Geometry: final body of the model. Coordinates: model frame, mm. Face numbers are marked on the shaded views. A direction names the side the tool comes from. Give positions to 0.01 mm unless a question says otherwise; leave off trailing zeros. Loops run counter-clockwise (first coordinate to the right, second up) from the corner with the lowest first, then second, coordinate; pieces in that order, holes last.
1. Section C-C, the plane x = -1.5. Output: boundary loops of the cut face in (y, z) (3 decimals), then the cut area to 3 significant figures.
2. Draft query along X for the marked faces 1, 2, 3 and 4. Return one class per face: +X half, -X half, draft (parallel to the pull), parting line (faces both ways), or undercut.
3. Access query for the marked faces 5, 6 and 7. Directions: +Z, -Z, +X, -X, +Y, -Y. A direction counts if a zero-diameter tool reaches every point of the face in a straight line with its end or side. Return the directions, or none.
4. Section D-D, the plane z = -3.25. Output: boundary loops of the cut face in (x, y) (3 decimals).
5. First-contact query: P1, Ø1, axis at x = -6, y = 3.5, coming from the -Z side; P2, Ø1, axis at y = 3.5, z = -7.5, coming from the -X side; P3, Ø2, axis at x = -1, z = -7, coming from the +Y side; P4, Ø0.5, axis at x = -5, z = -0.5, coming from the +Y side. Flat tips, straight axial feed; report the tip coordinate or a pass-through.
6. Section B-B, the plane z = -7.75. Output: boundary loops of the cut face in (x, y).
7. Material intervals for line 1 along Z through (x, y) = (-5.25, 4.5); line 2 along X through (y, z) = (1.85, -9.25); line 3 along X through (y, z) = (0.3, -9), sorted ascending.
8. Section A-A, the plane y = 4.5. Output: boundary loops of the cut face in (x, z).
Autodesk Inventor part; units mm, degrees
ref_plane "YZ Plane" through (0, 0, 0) normal (1, 0, 0) x (0, 1, 0)
ref_plane "XZ Plane" through (0, 0, 0) normal (0, 1, 0) x (-1, 0, 0)
ref_plane "XY Plane" through (0, 0, 0) normal (0, 0, 1) x (1, 0, 0)
sketch "Sketch1" plane through (0, 0, 0) normal (0, 1, 0) x (-1, 0, 0)
  line L0 (0, 0) -> (8.89, 0)
  line L1 (8.89, 0) -> (8.89, -10.16)
  line L2 (8.89, -10.16) -> (0, -10.16)
  line L3 (0, -10.16) -> (0, 0)
  dimension "d0" = 8.89
  dimension "d1" = 10.16
extrude "Extrusion1" add sketch "Sketch1" along normal blind 2.54
sketch "Sketch5" plane through (0, 2.54, 0) normal (0, 1, 0) x (1, 0, 0)
  line L0 (-8.89, 0) -> (0, 0)
  line L1 (0, 0) -> (0, 10.16)
  line L2 (0, 10.16) -> (-8.89, 10.16)
  line L3 (-8.89, 10.16) -> (-8.89, 0)
  line L4 (0, 0) -> (-8.89, 0)
  line L5 (-5.7785, 0) -> (-6.6294, 0.9271)
  line L6 (-6.6294, 0.9271) -> (-6.6294, 1.6764)
  line L7 (-6.6294, 1.6764) -> (-2.2606, 1.6764)
  line L8 (-2.2606, 1.6764) -> (-2.2606, 0.9271)
  line L9 (-2.2606, 0.9271) -> (-3.1115, 0)
  line L10 (-8.89, 0) -> (-8.89, 10.16)
  line L11 (-8.89, 3.81) -> (0, 3.81)
  point P0 (-4.445, 1.6764)
  point P1 (-4.445, 3.81)
  dimension "d19" = 2.667
  dimension "d20" = 4.3688
  dimension "d21" = 0.9271
  dimension "d23" = 1.6764
  dimension "d24" = 3.81
extrude "Extrusion4" add sketch "Sketch5" along normal blind 3.175 contours L3 L11 L1 L0 L9 L8 L7 L6 L5
sketch "Sketch6" plane through (0, 2.54, 0) normal (0, 1, 0) x (1, 0, 0)
  line L0 (-3.1115, 0) -> (-2.2606, 0.9271)
  line L1 (-2.2606, 0.9271) -> (-2.2606, 1.6764)
  line L2 (-2.2606, 1.6764) -> (-6.6294, 1.6764)
  line L3 (-6.6294, 1.6764) -> (-6.6294, 0.9271)
  line L4 (-6.6294, 0.9271) -> (-5.7785, 0)
  line L5 (-5.7785, 0) -> (-3.1115, 0)
  point P0 (0, 0)
extrude "Extrusion5" cut sketch "Sketch6" against normal blind 1.016
fillet "Fillet3" radius 1.27 6 edges at (-8.89, 1.27, -10.16) (0, 1.27, -10.16) (-8.89, 2.8575, 0) (-8.89, 4.1275, -3.81) (0, 4.1275, -3.81) (0, 2.8575, 0)
sketch "Sketch8" plane through (0, 2.54, 0) normal (0, 1, 0) x (1, 0, 0)
  line L0 (-7.62, 10.16) -> (-1.27, 10.16)
  line L1 (-6.1595, 10.16) -> (-6.1595, 7.874)
  line L2 (-2.7305, 10.16) -> (-2.7305, 7.874)
  arc A0 (-6.1595, 7.874) -> (-2.7305, 7.874) centre (-4.445, 7.874) ccw
  point P0 (0, 0)
  point P1 (-4.445, 10.16)
  dimension "d37" = 3.429
  dimension "d38" = 2.286
extrude "Extrusion7" cut sketch "Sketch8" against normal blind 25.4
fillet "Fillet4" radius 1.016 2 edges at (-2.7305, 1.27, -10.16) (-6.1595, 1.27, -10.16)
properties part number "HallEffectSpoolSensorMount3" material "ABS Plastic"
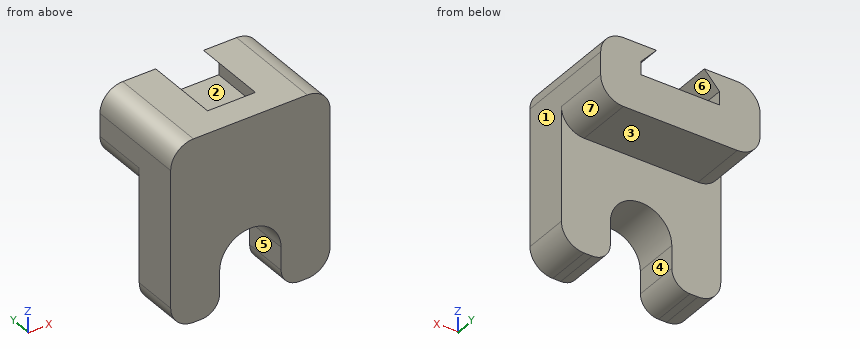
Answers below:
1. outline: (0, -10.16) - (2.54, -10.16) - (2.54, -3.81) - (5.715, -3.81) - (5.715, 0) - (0, 0) - close
1. area: 37.9 mm2
2. face 1: +X half
2. face 2: undercut
2. face 3: draft
2. face 4: undercut
3. face 5: -Z, +Y, -Y
3. face 6: +Y
3. face 7: -Z, +X, +Y
4. outline: (-8.89, 0) - (0, 0) - (0, 2.54) - (-0.217, 2.54) - (-0.217, 5.715) - (-8.673, 5.715) - (-8.673, 2.54) - (-8.89, 2.54) - close
5. P1: stops at z = -3.81
5. P2: passes through
5. P3: stops at y = 2.54
5. P4: stops at y = 1.52
6. outline: (-8.89, 0) - (-6.16, 0) - (-6.16, 2.54) - (-8.89, 2.54) - close; (-2.73, 0) - (0, 0) - (0, 2.54) - (-2.73, 2.54) - close
7. line 1: z = -3.81 to -1.68
7. line 2: x = -8.84 to -6.17, -2.72 to -0.05
7. line 3: x = -8.89 to -6.16, -2.73 to 0
8. outline: (-8.89, -2.54) arc R1.27 ccw to (-7.62, -3.81) - (-1.27, -3.81) arc R1.27 ccw to (0, -2.54) - (0, -1.27) arc R1.27 ccw to (-1.27, 0) - (-3.11, 0) - (-2.26, -0.93) - (-2.26, -1.68) - (-6.63, -1.68) - (-6.63, -0.93) - (-5.78, 0) - (-7.62, 0) arc R1.27 ccw to (-8.89, -1.27) - close
